from build123d import *
from OCP.BRepFilletAPI import BRepFilletAPI_MakeChamfer

# Parameters (mm, degrees)
SKETCH1_R               = 4.765
BOSS_EXTRUDE1_DEPTH     = 9.5
CHAMFER1_SIZE           = 2.54
CHAMFER1_SIZE2          = 7.62
CHAMFER3_SIZE           = 7.62
CHAMFER3_SIZE2          = 2.54
CUT_EXTRUDE2_DEPTH      = 32.701013029
CUT_EXTRUDE2_DEPTH_BACK = 32.701013029
SKETCH3_W               = 9.53
SKETCH3_H               = 9.53
CUT_EXTRUDE5_DEPTH      = 50
SKETCH4_R               = 1.59
CUT_EXTRUDE6_DEPTH      = 50


with BuildPart() as part:
    # Sketch1 → Boss-Extrude1 (new, symmetric)
    with BuildSketch(Plane(origin=(0, 0, 0), x_dir=(0, 0, -1), z_dir=(1, 0, 0))):
        with BuildLine():
            Line((0, 9.908259288), (-22.225, 9.908259288))
            Line((-22.225, 9.908259288), (-22.225, 4.908259288))
            Line((-22.225, 4.908259288), (-9.871538087, -0.852254607))
            ThreePointArc((-9.871538087, -0.852254607), (-6.033040367, -7.859772645), (1.728564082, -9.75631428))
            Line((1.728564082, -9.75631428), (28.574999999, -4.999826991))
            Line((28.574999999, -4.999826991), (28.574999999, 0.000173009))
            Line((28.574999999, 0.000173009), (9.908259287, 5.999e-05))
            ThreePointArc((9.908259287, 5.999e-05), (7.006176122, 7.006218542), (0, 9.908259288))
        make_face()
        Circle(SKETCH1_R, mode=Mode.SUBTRACT)
    extrude(amount=BOSS_EXTRUDE1_DEPTH, both=True)

    # Chamfer1: one chamfer whose edges measure the first distance from different faces: ONE call of the kernel's chamfer builder (chamfer() names one face for all edges)
    chamfer1_edges_1 = [part.edges().sort_by_distance(p)[0] for p in [
        (9.5, 7.408259288, 22.225),
    ]]
    chamfer1_side_1 = [part.faces().sort_by_distance(p)[0] for p in [
        (0, 7.408259288, 22.225),
    ]]
    chamfer1_edges_2 = [part.edges().sort_by_distance(p)[0] for p in [
        (9.5, -2.499826991, -28.574999999),
    ]]
    chamfer1_side_2 = [part.faces().sort_by_distance(p)[0] for p in [
        (0, -2.499826991, -28.574999999),
    ]]
    chamfer1 = BRepFilletAPI_MakeChamfer(part.part.solid().wrapped)
    for e in chamfer1_edges_1:
        chamfer1.Add(CHAMFER1_SIZE, CHAMFER1_SIZE2, e.wrapped, chamfer1_side_1[0].wrapped)  # the first distance lies on this face
    for e in chamfer1_edges_2:
        chamfer1.Add(CHAMFER1_SIZE, CHAMFER1_SIZE2, e.wrapped, chamfer1_side_2[0].wrapped)  # the first distance lies on this face
    add(Compound.cast(chamfer1.Shape()), mode=Mode.REPLACE)

    # Chamfer3
    chamfer3_edges = [part.edges().sort_by_distance(p)[0] for p in [
        (-9.5, 7.408259288, 22.225),
        (-9.5, -2.499826991, -28.574999999),
    ]]
    chamfer3_side = [part.faces().sort_by_distance(p)[0] for p in [
        (-9.5, 9.362976388, 11.1125),
    ]]
    chamfer(chamfer3_edges, length=CHAMFER3_SIZE, length2=CHAMFER3_SIZE2, reference=chamfer3_side[0])

    # Sketch2 → Cut-Extrude2 (cut, two sides: drawn at the far end of the back side and taken through both)
    with BuildSketch(Plane(origin=(0, 0, 0), x_dir=(1, 0, 0), z_dir=(0, 1, 0)).offset(-CUT_EXTRUDE2_DEPTH_BACK)):
        with BuildLine():
            Line((-5.08, -3.81), (-5.08, 6.35))
            ThreePointArc((-5.08, 6.35), (0, 11.43), (5.08, 6.35))
            Line((5.08, 6.35), (5.08, -3.81))
            ThreePointArc((5.08, -3.81), (0, -8.89), (-5.08, -3.81))
        make_face()
    extrude(amount=CUT_EXTRUDE2_DEPTH + CUT_EXTRUDE2_DEPTH_BACK, mode=Mode.SUBTRACT)

    # Sketch3 → Cut-Extrude5 (cut, symmetric)
    with BuildSketch(Plane(origin=(0, 0, 0), x_dir=(1, 0, 0), z_dir=(0, 0.9999999999816713, 6.054544672321462e-06))):
        Polygon((-4.765, -22.22494001), (-4.765, -26.288329998), (4.765, -26.288329998), (4.765, -22.22494001), (4.765, -12.69494001), (-4.765, -12.69494001), align=None)
        with Locations((0, 23.81)):
            Rectangle(SKETCH3_W, SKETCH3_H)
    extrude(amount=CUT_EXTRUDE5_DEPTH, both=True, mode=Mode.SUBTRACT)

    # Sketch4 → Cut-Extrude6 (cut, symmetric)
    with BuildSketch(Plane(origin=(0, 0, 0), x_dir=(0, 0, -1), z_dir=(1, 0, 0))):
        with Locations((26.034999999, -2.53984237)):
            Circle(SKETCH4_R)
        with Locations(Location((-19.685, 7.368259288, 0), (0, 0, 180))):
            Circle(SKETCH4_R)
    extrude(amount=CUT_EXTRUDE6_DEPTH, both=True, mode=Mode.SUBTRACT)


solid = part.part
Check sheet for the modelled part. Datum: model origin and axes. Units: mm. A direction names the side the tool comes from. Give positions to 0.01 mm unless a question says otherwise; leave off trailing zeros. Loops run counter-clockwise (first coordinate to the right, second up) from the corner with the lowest first, then second, coordinate; pieces in that order, holes last. Notation, with made-up numbers: M 29.25,22 L 36.25,22 A27 cw 36.25,48 Z; hole C 63.25,75 d9. An arc over 180 degrees is marked long. Return JSON: item names as keys, results as strings. Group by question number.
1. Cross-section at D-D on z = 6.5. Record the boundary of the cut face in (x, y).
2. Mould release check, pull along X, two halves, no side actions. Record for faces 4 (the flat face through (5.08, -2, -5)), 5 (the cylindrical face through (-6.148, -2.47, -24.447)), 6 (the flat face through (8.53, -3.22, -23.86)): released by +X, released by -X, zero draft, split by the parting line, or undercut.
3. Go/stop test with flat-tipped pins: pin 1 (2 mm diameter, centred on x = -2, y = -3.5, fed in from -Z) (3 decimals); pin 2 (3 mm diameter, centred on x = -3.5, z = -18, fed in from +Y); pin 3 (3.5 mm diameter, centred on y = -2.54, z = -26.03, fed in from -X); pin 4 (10.5 mm diameter, centred on y = 4, z = 15, fed in from +X). Record where each tip stops, or that it passes through.
4. Tool access check on faces 1 (the flat face through (4.765, -3, -23)), 2 (the flat face through (-8.494, -3.219, -23.972)), 3 (the flat face through (-5.08, -2, -5)). Record the directions out of +Z, -Z, +X, -X, +Y, -Y that give a thin tool (end or side, any length) a straight path to the whole face; none if there is none.
5. Cross-section at A-A on z = -20. Record the boundary of the cut face in (x, y) (3 decimals).
6. Cross-section at B-B on x = -0.5. Record the boundary of the cut face in (y, z) (3 decimals), plus the area to 4 significant figures.
7. Thickness scan on L1, parallel to Y at x = -6.95, z = 0 (3 decimals); L2, parallel to X at y = 1.75, z = -5; L3, parallel to X at y = 5.5, z = 13 (3 decimals). Record the ranges inside material, lowest first.
8. Cross-section at C-C on y = -2. Record the boundary of the cut face in (x, z) (3 decimals).
Return value:
{
 "1": {"outline": "M -9.5,-7.48 L -4.31,-7.48 L -4.31,9.91 L -9.5,9.91 Z; M 4.31,-7.48 L 9.5,-7.48 L 9.5,9.91 L 4.31,9.91 Z"},
 "2": {"face 4": "undercut", "face 5": "zero draft", "face 6": "released by +X"},
 "3": {"pin 1": "z = -19.045", "pin 2": "y = 0", "pin 3": "x = -8.39", "pin 4": "x = 9.5"},
 "4": {"face 1": "-Z, +Y, -Y", "face 2": "-Z, -X, +Y, -Y", "face 3": "+Y, -Y"},
 "5": {"outline": "M -9.5,-6.519 L -4.765,-6.519 L -4.765,0 L -9.5,0 Z; M 4.765,-6.519 L 9.5,-6.519 L 9.5,0 L 4.765,0 Z"},
 "6": {"outline": "M -8.042,-11.405 L -6.688,-19.045 L 0,-19.045 L 0,-11.405 Z; M -4.425,8.865 L 9.908,8.865 L 9.908,12.695 L 0.464,12.695 L -0.852,9.872 A9.908 ccw Z", "area": "97.85 mm^2"},
 "7": {"L1": "-9.908 to -4.765, 4.765 to 9.908", "L2": "-9.5 to -5.08, 5.08 to 9.5", "L3": "-9.5 to -4.765, 4.765 to 9.5"},
 "8": {"outline": "M -9.5,-20.955 L -8.305,-24.539 L -4.765,-24.539 L -4.765,-19.045 L 4.765,-19.045 L 4.765,-24.539 L 8.305,-24.539 L 9.5,-20.955 L 9.5,-4.325 L 5.08,-4.325 L 5.08,-6.35 A5.08 cw -5.08,-6.35 L -5.08,-4.325 L -9.5,-4.325 Z; M -9.5,4.325 L -5.054,4.325 A5.08 cw 5.054,4.325 L 9.5,4.325 L 9.5,9.704 L -9.5,9.704 Z; M -7.308,-27.531 L -6.96,-28.575 L -4.765,-28.575 L -4.765,-27.531 Z; M 4.765,-28.575 L 6.96,-28.575 L 7.308,-27.531 L 4.765,-27.531 Z"}
}
